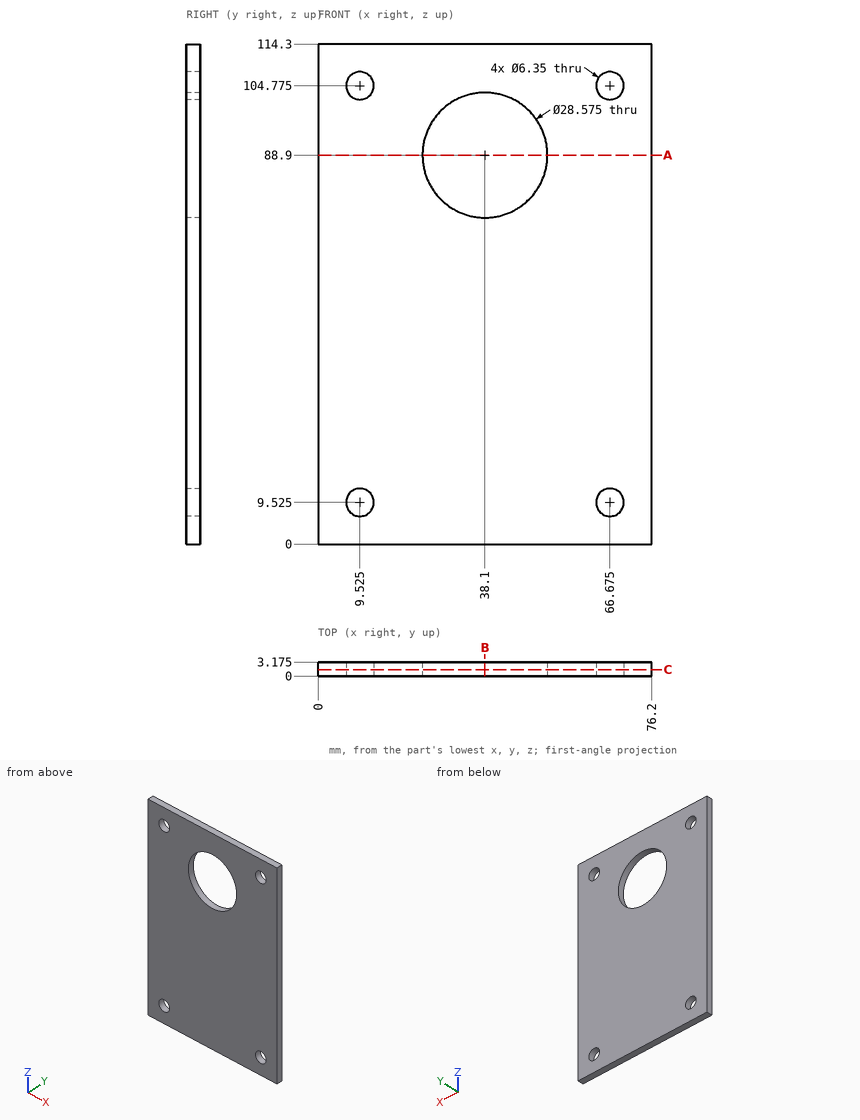
Study the drawing (mm; zero at the part's minimum x, y, z) and answer. Round coordinates to 2 decimals unless told otherwise and drop trailing zeros. Write each loop counter-clockwise with the first axis right and the second up, starting at its lowest first coordinate (ties: lowest second). Pieces come first, ordered by that corner, then holes.
1) A cutting plane is placed at C-C (y = 1.45). Give the number of separate pieces and of enclosed holes in the cut face, plus the area to 3 significant figures.
2) Given pin 1 Ø10 at (x, z) = (9.525, 104.775) entering from +Y (3 decimals), flat-ended and moving along its own axis, determine where the tip first touches the part or whether it passes through.
3) A cutting plane is placed at A-A (z = 88.9). Give the vertices of the cut face in (x, y) (1 decimal), plus the area to 3 significant figures.
4) A cutting plane is placed at B-B (x = 38.1). Give the vertices of the cut face in (y, z) (1 decimal).
5) Straight lines are drawn through the part: line 1 (Z direction, x = 65, y = 0.7); line 2 (Z direction, x = 10.5, y = 0.95); line 3 (X direction, y = 2.55, z = 88.9). For each, find the intervals that lie inside material, in ascending order.
Completed:
1. separate pieces: 1
1. enclosed holes: 5
1. area: 7,940 mm2
2. pin 1: stops at y = 3.175
3. outline: (0, 0) - (23.8, 0) - (23.8, 3.2) - (0, 3.2) - close; (52.4, 0) - (76.2, 0) - (76.2, 3.2) - (52.4, 3.2) - close
3. area: 151 mm2
4. outline: (0, 0) - (3.2, 0) - (3.2, 74.6) - (0, 74.6) - close; (0, 103.2) - (3.2, 103.2) - (3.2, 114.3) - (0, 114.3) - close
5. line 1: z = 0 to 6.83, 12.22 to 102.08, 107.47 to 114.3
5. line 2: z = 0 to 6.5, 12.55 to 101.75, 107.8 to 114.3
5. line 3: x = 0 to 23.81, 52.39 to 76.2
